```python
from build123d import *

# Parameters (mm, degrees)
SKETCH2_R          = 13.335
EXTRUDE1_DEPTH     = 17.78
EXTRUDE1_DRAFT     = 1.5
CHAMFER1_SIZE      = 1.366157143
CHAMFER1_SIZE2     = 1.403374095
EXTRUDE2_DEPTH     = 6.096
SKETCH6_R          = 6.858
CUT_EXTRUDE1_DEPTH = 28.353582774
CUT_EXTRUDE1_DRAFT = 1.5
SKETCH12_OUTSIDE_W = 152.316
SKETCH12_OUTSIDE_H = 155.804
SKETCH12_OUTSIDE_R = 13.462
CUT_EXTRUDE6_DEPTH = 32.656807587
CUT_EXTRUDE6_DRAFT = -60
SKETCH13_OUTSIDE_W = 137.41
SKETCH13_OUTSIDE_H = 140.898
SKETCH13_OUTSIDE_R = 13.462
CUT_EXTRUDE7_DEPTH = 28.353582774
CUT_EXTRUDE7_DRAFT = -60
SKETCH15_R         = 6.858
CUT_EXTRUDE8_DEPTH = 28.353582774


with BuildPart() as part:
    # Sketch2 → Extrude1 (with draft: the straight prism first)
    with BuildSketch(Plane(origin=(11.938, 0, 0), x_dir=(0, 0, -1), z_dir=(1, 0, 0))):
        Circle(SKETCH2_R)
    extrude(amount=-EXTRUDE1_DEPTH)
    # Extrude1: the draft: its side faces are tilted about the plane it starts from
    extrude1_sides = [part.faces().sort_by_distance(p)[0] for p in [
        (3.048, 0, 13.335),
    ]]
    draft(extrude1_sides, Plane(origin=(11.938, 0, 0), x_dir=(0, 0, -1), z_dir=(1, 0, 0)), EXTRUDE1_DRAFT)

    # Chamfer1
    chamfer1_edges = [part.edges().sort_by_distance(p)[0] for p in [
        (11.938, 0, 13.335),
    ]]
    chamfer1_side = [part.faces().sort_by_distance(p)[0] for p in [
        (3.048, 0, 13.567792843),
    ]]
    chamfer(chamfer1_edges, length=CHAMFER1_SIZE, length2=CHAMFER1_SIZE2, reference=chamfer1_side[0])

    # Sketch5 → Extrude2 (add)
    with BuildSketch(Plane.ZY.offset(5.842)):
        Polygon((0, 15.544578648), (-13.462, 7.772289324), (-13.462, -7.772289324), (0, -15.544578648), (13.462, -7.772289324), (13.462, 7.772289324), align=None)
    extrude(amount=EXTRUDE2_DEPTH)


with BuildPart() as cut_extrude1_tool:
    # Sketch6 → Cut-Extrude1 (with draft: the straight prism first)
    with BuildSketch(Plane(origin=(-5.842, 0, 0), x_dir=(0, 0, -1), z_dir=(1, 0, 0))):
        Circle(SKETCH6_R)
    extrude(amount=-CUT_EXTRUDE1_DEPTH)
    # Cut-Extrude1: the draft: its side faces are tilted about the plane it starts from
    cut_extrude1_sides = [cut_extrude1_tool.faces().sort_by_distance(p)[0] for p in [
        (-20.018791387, 0, 6.858),
    ]]
    draft(cut_extrude1_sides, Plane(origin=(-5.842, 0, 0), x_dir=(0, 0, -1), z_dir=(1, 0, 0)), CUT_EXTRUDE1_DRAFT)


with BuildPart() as part_1:
    add(part.part)

    # Cut-Extrude1: cut by cut_extrude1_tool
    add(cut_extrude1_tool.part, mode=Mode.SUBTRACT)

    # Cut-Extrude4 cone 1 section (through the dimple's axis) → Cut-Extrude4 (revolve, cut)
    with BuildSketch(Plane(origin=(-11.938, 0, 0), x_dir=(0, 0, 1), z_dir=(0, 1, 0))):
        Polygon((0, 0), (7.017629378, 0), (0, 7.017629378), align=None)
    revolve(axis=Axis((-11.938, 0, 0), (1, 0, 0)), mode=Mode.SUBTRACT)


with BuildPart() as cut_extrude6_tool:
    # Sketch12 outside → Cut-Extrude6 (with draft: the straight prism first)
    with BuildSketch(Plane.ZY.offset(11.938)):
        Rectangle(SKETCH12_OUTSIDE_W, SKETCH12_OUTSIDE_H)
        Circle(SKETCH12_OUTSIDE_R, mode=Mode.SUBTRACT)
    extrude(amount=-CUT_EXTRUDE6_DEPTH)
    # Cut-Extrude6: the draft: its side faces are tilted about the plane it starts from
    cut_extrude6_sides = [cut_extrude6_tool.faces().sort_by_distance(p)[0] for p in [
        (4.390403793, -77.902, 0),
        (4.390403793, 0, 76.158),
        (4.390403793, 77.902, 0),
        (4.390403793, 0, -76.158),
        (4.390403793, 0, -13.462),
    ]]
    draft(cut_extrude6_sides, Plane.ZY.offset(11.938), CUT_EXTRUDE6_DRAFT)


with BuildPart() as part_2:
    add(part_1.part)

    # Cut-Extrude6: cut by cut_extrude6_tool
    add(cut_extrude6_tool.part, mode=Mode.SUBTRACT)


with BuildPart() as cut_extrude7_tool:
    # Sketch13 outside → Cut-Extrude7 (with draft: the straight prism first)
    with BuildSketch(Plane(origin=(-5.842, 0, 0), x_dir=(0, 0, -1), z_dir=(1, 0, 0))):
        Rectangle(SKETCH13_OUTSIDE_W, SKETCH13_OUTSIDE_H)
        Circle(SKETCH13_OUTSIDE_R, mode=Mode.SUBTRACT)
    extrude(amount=-CUT_EXTRUDE7_DEPTH)
    # Cut-Extrude7: the draft: its side faces are tilted about the plane it starts from
    cut_extrude7_sides = [cut_extrude7_tool.faces().sort_by_distance(p)[0] for p in [
        (-20.018791387, -70.449, 0),
        (-20.018791387, 0, -68.705),
        (-20.018791387, 70.449, 0),
        (-20.018791387, 0, 68.705),
        (-20.018791387, 0, 13.462),
    ]]
    draft(cut_extrude7_sides, Plane(origin=(-5.842, 0, 0), x_dir=(0, 0, -1), z_dir=(1, 0, 0)), CUT_EXTRUDE7_DRAFT)


with BuildPart() as part_3:
    add(part_2.part)

    # Cut-Extrude7: cut by cut_extrude7_tool
    add(cut_extrude7_tool.part, mode=Mode.SUBTRACT)

    # Sketch15 → Cut-Extrude8 (cut, through all)
    with BuildSketch(Plane.ZY.offset(5.842)):
        Circle(SKETCH15_R)
    extrude(amount=-CUT_EXTRUDE8_DEPTH, mode=Mode.SUBTRACT)


solid = part_3.part
```
Check sheet for the modelled part. Datum: model origin and axes. Units: mm. A direction names the side the tool comes from. Round coordinates to 2 decimals unless told otherwise and drop trailing zeros. Loops run counter-clockwise (first coordinate to the right, second up) from the corner with the lowest first, then second, coordinate; pieces in that order, holes last. Notation, with made-up numbers: (29.5, 81.5) - (64.5, 81.5) arc R13 cw to (64.5, 102.5) - close; hole circle Ø1 at (-38, 61). An arc over 180 degrees is marked (long way). Answer as a JSON object with one key per item and string values. Group by question number.
Q1. Sectioned sample at B-B, the plane x = 0.75. Enter the section's corners in (y, z), plus the area to 3 significant figures.
Q2. Scan lines: line 1 along Y through (x, z) = (-1.5, 0); line 2 along Z through (x, y) = (3.5, -3); line 3 along Y through (x, z) = (6, 6). Record each from-to range of solid material in increasing order. Write a range as [from, to].
Q3. Mould release check, pull along X, two halves, no side actions. Record for faces 1 (the face through (-6.13, 7.01, 12.07)), 2 (the face through (-11.65, 7.01, -12.07)), 3 (the face through (-9, 0, -13.462)): released by +X, released by -X, zero draft, split by the parting line, or undercut.
Q4. Sectioned sample at A-A, the plane x = 4.5. Enter the section's corners in (y, z).
Q5. Set-up check for faces 4 (the face through (-8.85, 11.71, -6.64)), 5 (the face through (-5.842, -12.2, -6.1)), 6 (the face through (-8.85, -11.71, 6.64)): record each of +Z, -Z, +X, -X, +Y, -Y from which the full face is reachable in a straight line by a thin tool's end or side.
Q6. Gauge pin test, flat ends, axial feed: P1, Ø8, axis at x = 6, z = 9, coming from the -Y side; P2, Ø10, axis at x = -9.5, z = 2.5, coming from the +Y side; P3, Ø6, axis at x = -2, y = -1.5, coming from the -Z side; P4, Ø3, axis at x = -8, y = 1, coming from the +Z side. Record the tip position at first contact, or that the pin passes through.
Solution:
{
 "1": {"outline": "circle Ø27.26 at (0, 0); hole circle Ø13.72 at (0, 0)", "area": "436 mm²"},
 "2": {"line 1": "y = [-13.69, -6.86], [6.86, 13.69]", "line 2": "z = [-13.22, -6.17], [6.17, 13.22]", "line 3": "y = [-12.08, -3.32], [3.32, 12.08]"},
 "3": {"face 1": "undercut", "face 2": "released by -X", "face 3": "zero draft"},
 "4": {"outline": "circle Ø27.06 at (0, 0); hole circle Ø13.72 at (0, 0)"},
 "5": {"face 4": "-Z, -X, +Y", "face 5": "none", "face 6": "+Z, -X, -Y"},
 "6": {"P1": "stops at y = -12.53", "P2": "stops at y = 15.54", "P3": "stops at z = -13.77", "P4": "stops at z = 13.46"}
}
